Verification items for the finished model (mm, model axes). A direction names the side the tool comes from. Round coordinates to 2 decimals unless told otherwise and drop trailing zeros. Write each loop counter-clockwise with the first axis right and the second up, starting at its lowest first coordinate (ties: lowest second). Pieces come first, ordered by that corner, then holes. Notation, with made-up numbers: M 10.25,0.25 L 52.25,0.25 A19 cw 52.25,37.25 Z; hole C 62.25,33.5 d10. An arc over 180 degrees is marked long. One line per question, with ' | ' between items.
from build123d import *

# Parameters (mm, degrees)
SKETCH_1_W          = 24
SKETCH_1_H          = 11
EXTRUDE_1_DEPTH     = 3.2
SKETCH_2_W          = 20
SKETCH_2_H          = 3
CUT_EXTRUDE_1_DEPTH = 2.8
SKETCH_3_W          = 3
SKETCH_3_H          = 7.6
CUT_EXTRUDE_2_DEPTH = 2.8
FILLET_1_R          = 2
FILLET_2_R          = 1


with BuildPart() as part:
    # ｽｹｯﾁ1 → ﾎﾞｽ - 押し出し1 (new body)
    with BuildSketch(Plane.XY):
        with Locations((11.314402496, 5.5)):
            Rectangle(SKETCH_1_W, SKETCH_1_H)
    extrude(amount=EXTRUDE_1_DEPTH)

    # ｽｹｯﾁ2 → ｶｯﾄ - 押し出し1 (cut)
    with BuildSketch(Plane.XY.offset(3.2)):
        with Locations((11.314402496, 9.1)):
            Rectangle(SKETCH_2_W, SKETCH_2_H)
    extrude(amount=-CUT_EXTRUDE_1_DEPTH, mode=Mode.SUBTRACT)

    # ｽｹｯﾁ3 → ｶｯﾄ - 押し出し2 (cut)
    with BuildSketch(Plane.XY.offset(3.2)):
        with Locations((19.814402496, 3.8)):
            Rectangle(SKETCH_3_W, SKETCH_3_H)
        with Locations((2.814402496, 3.8)):
            Rectangle(SKETCH_3_W, SKETCH_3_H)
    extrude(amount=-CUT_EXTRUDE_2_DEPTH, mode=Mode.SUBTRACT)

    # ﾌｨﾚｯﾄ1
    fillet_1_edges = [part.edges().sort_by_distance(p)[0] for p in [
        (-0.685597504, 11, 1.6),
        (23.314402496, 11, 1.6),
    ]]
    fillet(fillet_1_edges, radius=FILLET_1_R)

    # ﾌｨﾚｯﾄ2
    fillet_2_edges = [part.edges().sort_by_distance(p)[0] for p in [
        (1.314402496, 10.6, 1.8),
        (21.314402496, 10.6, 1.8),
    ]]
    fillet(fillet_2_edges, radius=FILLET_2_R)


solid = part.part
1. Thickness scan on line 1 (X direction, y = 7.5, z = 2.5); line 2 (Y direction, x = 13.5, z = 1); line 3 (X direction, y = 7.75, z = 1.7). Record the ranges inside material, lowest first.
Results:
line 1: x = -0.69 to 1.31, 4.31 to 18.31, 21.31 to 23.31 | line 2: y = 0 to 7.6, 10.6 to 11 | line 3: x = -0.69 to 1.31, 21.31 to 23.31
2. Section check A-A, the plane z = 2.45. Record the cut outline in (x, y), then the cut area to 3 significant figures.
Results:
outline: M -0.69,0 L 1.31,0 L 1.31,9.6 A1 cw 2.31,10.6 L 20.31,10.6 A1 cw 21.31,9.6 L 21.31,0 L 23.31,0 L 23.31,9 A2 ccw 21.31,11 L 1.31,11 A2 ccw -0.69,9 Z; M 4.31,0 L 18.31,0 L 18.31,7.6 L 4.31,7.6 Z | area: 157 mm2
3. Section check B-B, the plane x = 13.25. Record the cut outline in (y, z).
Results:
outline: M 0,0 L 11,0 L 11,3.2 L 10.6,3.2 L 10.6,0.4 L 7.6,0.4 L 7.6,3.2 L 0,3.2 Z
4. Section check D-D, the plane y = 8.25. Record the cut outline in (x, z).
Results:
outline: M -0.69,0 L 23.31,0 L 23.31,3.2 L 21.31,3.2 L 21.31,0.4 L 1.31,0.4 L 1.31,3.2 L -0.69,3.2 Z
5. Mould release check, pull along X, two halves, no side actions. Record for faces 4 (the face through (-0.115, 10.399, 1.622)), 5 (the face through (18.314, 4, 2)), 6 (the face through (11, 11, 2)): pulls with the +X half, pulls with the -X half, needs draft (parallel to the pull), parting line crosses it, or undercut.
Results:
face 4: pulls with the -X half | face 5: undercut | face 6: needs draft
6. Section check C-C, the plane y = 3.5. Record the cut outline in (x, z), then the cut area to 3 significant figures.
Results:
outline: M -0.69,0 L 23.31,0 L 23.31,3.2 L 21.31,3.2 L 21.31,0.4 L 18.31,0.4 L 18.31,3.2 L 4.31,3.2 L 4.31,0.4 L 1.31,0.4 L 1.31,3.2 L -0.69,3.2 Z | area: 60.0 mm2
7. Tool access check on faces 1 (the face through (11, 0, 2)), 2 (the face through (11, 7.6, 2)), 3 (the face through (21.03, 10.3, 1.78)). Record the directions out of +Z, -Z, +X, -X, +Y, -Y that give a thin tool (end or side, any length) a straight path to the whole face; none if there is none.
Results:
face 1: +Z, -Z, +X, -X, -Y | face 2: +Z | face 3: +Z, -Y
